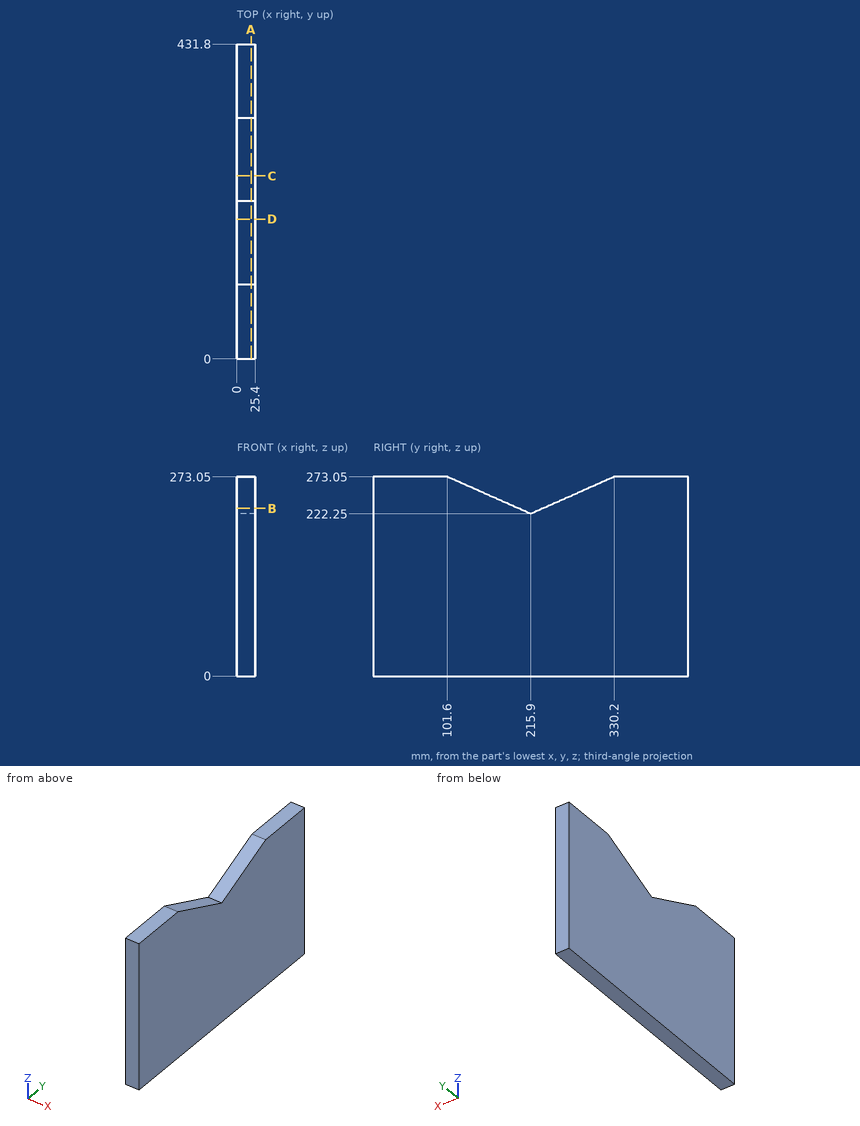
Study the drawing (mm; zero at the part's minimum x, y, z) and answer. Coordinates: 2 decimals unless noted, no trailing zeros. Write each loop counter-clockwise with the first axis right and the second up, starting at its lowest first coordinate (ties: lowest second). Pieces come first, ordered by that corner, then holes.
Q1. A cutting plane is placed at D-D, the plane y = 191.5. Give the vertices of the cut face in (x, z).
Q2. A cutting plane is placed at A-A, the plane x = 19.5. Give the vertices of the cut face in (y, z).
Q3. A cutting plane is placed at B-B, the plane z = 230. Give the vertices of the cut face in (x, y), then the cut area to 3 significant figures.
Q4. A cutting plane is placed at C-C, the plane y = 251. Give the vertices of the cut face in (x, z).
Q5. Each of these flat-tipped pins is pushed along its axis until it touches: pin 1 Ø3 at (x, y) = (3, 339) entering from -Z; pin 2 Ø6 at (x, y) = (11.5, 183) entering from +Z; pin 3 Ø6 at (x, y) = (15, 217.5) entering from +Z; pin 4 Ø6 at (x, y) = (7, 116) entering from +Z. Where does it stop, or does it pass through?
Q6. Find the intervals of material crossed by line 1 (Y direction, x = 1.5, z = 243); line 2 (Y direction, x = 19.25, z = 231.5); line 3 (Z direction, x = 17.75, y = 261), in increasing order.
Findings below:
1. outline: (0, 0) - (25.4, 0) - (25.4, 233.09) - (0, 233.09) - close
2. outline: (0, 0) - (431.8, 0) - (431.8, 273.05) - (330.2, 273.05) - (215.9, 222.25) - (101.6, 273.05) - (0, 273.05) - close
3. outline: (0, 0) - (25.4, 0) - (25.4, 198.46) - (0, 198.46) - close; (0, 233.34) - (25.4, 233.34) - (25.4, 431.8) - (0, 431.8) - close
3. area: 10,100 mm2
4. outline: (0, 0) - (25.4, 0) - (25.4, 237.85) - (0, 237.85) - close
5. pin 1: stops at z = 0
5. pin 2: stops at z = 238.21
5. pin 3: stops at z = 224.29
5. pin 4: stops at z = 267.98
6. line 1: y = 0 to 169.21, 262.59 to 431.8
6. line 2: y = 0 to 195.09, 236.71 to 431.8
6. line 3: z = 0 to 242.29
